The listing builds one solid part. Answer for the finished solid, in the listing's coordinates (mm). Face numbers are marked on the shaded views. A direction names the side the tool comes from. Round coordinates to 2 decimals unless told otherwise and drop trailing zeros. Write each loop counter-clockwise with the first axis right and the second up, starting at its lowest first coordinate (ties: lowest second). Pieces come first, ordered by that corner, then holes.
Item 1: Find section D-D on x = 0.2. Give the vertices of the cut face in (y, z) (3 decimals).
Item 2: Each of these flat-tipped pins is pushed along its axis until it touches: pin 1 (0.8 mm diameter, centred on y = -0.5, z = 1, fed in from -X); pin 2 (0.8 mm diameter, centred on y = -2.5, z = 1, fed in from +X); pin 3 (0.8 mm diameter, centred on x = 1.5, z = 1, fed in from -Y). Where does it stop, or does it pass through?
Item 3: Find the intervals of material crossed by probe 1 along X at (y, z) = (-4.55, 1.25); probe 2 along X at (y, z) = (-2.25, -0.05); probe 3 along Y at (x, z) = (-1.95, 1.45), in increasing order.
Item 4: Find section B-B on z = 1.6. Give the vertices of the cut face in (x, y).
Item 5: Find section C-C on y = 0.5. Give the vertices of the cut face in (x, z) (3 decimals).
Item 6: Find section A-A on z = 0. Give the vertices of the cut face in (x, y), then the cut area to 3 significant figures.
Item 7: A tool of negligible diameter and unlimited length cuts with its end or side. For the marked faces 1, 2 and 3, from which of +Z, -Z, +X, -X, +Y, -Y can it reach the whole face along a straight path? Write none if from no direction.
```python
from build123d import *

# Parameters (mm, degrees)
SKETCH1_W                  = 1.5
SKETCH1_H                  = 0.75
BOSS_EXTRUDE1_DEPTH        = 1.875
BOSS_EXTRUDE1_DEPTH_BACK   = 0.625
FILLET1_R                  = 0.5
F_0_4_0_4_DIAMETER_HOLE1_D = 0.4


with BuildPart() as part:
    # Sketch1 → Boss-Extrude1 (new body, two sides)
    with BuildSketch(Plane.XY) as boss_extrude1_sk:
        Polygon((0.285769435, 0.25), (-1.464230565, 0.25), (-1.464230565, -4), (-1.464230565, -4.75), (0.285769435, -4.75), align=None)
        Polygon((-1.464230565, 2), (-1.464230565, 0.25), (0.285769435, 0.25), (1.535769435, 0.25), (1.535769435, 2), align=None)
        with Locations((-2.214230565, -4.375)):
            Rectangle(SKETCH1_W, SKETCH1_H)
    extrude(amount=BOSS_EXTRUDE1_DEPTH)
    extrude(boss_extrude1_sk.sketch, amount=-BOSS_EXTRUDE1_DEPTH_BACK)

    # Fillet1
    fillet1_edges = [part.edges().sort_by_distance(p)[0] for p in [
        (0.285769435, 0.25, 0.625),
        (-2.964230565, -4, 0.625),
        (-1.464230565, -4, 0.625),
        (0.285769435, -4.75, 0.625),
        (-1.464230565, 2, 0.625),
    ]]
    fillet(fillet1_edges, radius=FILLET1_R)

    # Ø0.4 (0.4) Diameter Hole1 (through all)
    with Locations(Plane(origin=(0, -4, 0), x_dir=(1, 0, 0), z_dir=(0, 1, 0))):
        with Locations((-2.214230565, 0), (-2.214230565, -1.25)):
            Hole(F_0_4_0_4_DIAMETER_HOLE1_D / 2)


solid = part.part
```
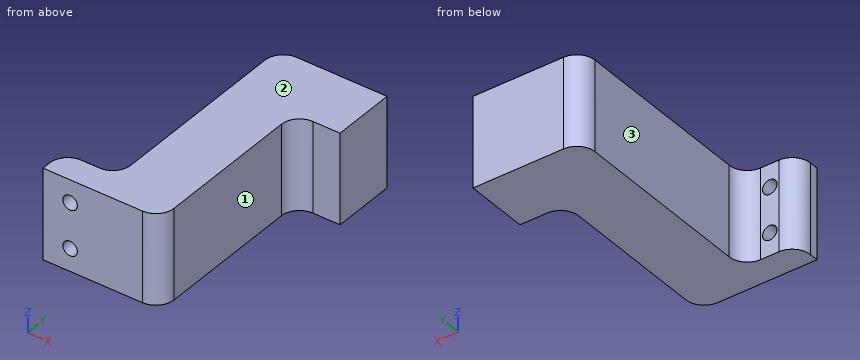
Check values:
1. outline: (-4.53, -0.625) - (2, -0.625) - (2, 1.875) - (-4.53, 1.875) - close
2. pin 1: stops at x = -1.46
2. pin 2: stops at x = 0.29
2. pin 3: stops at y = 0.25
3. probe 1: x = -2.96 to -2.41, -2.01 to 0.19
3. probe 2: x = -1.46 to 0.29
3. probe 3: y = -4.75 to -4
4. outline: (-2.96, -4.75) - (-0.21, -4.75) arc R0.5 ccw to (0.29, -4.25) - (0.29, -0.25) arc R0.5 cw to (0.79, 0.25) - (1.54, 0.25) - (1.54, 2) - (-0.96, 2) arc R0.5 ccw to (-1.46, 1.5) - (-1.46, -3.5) arc R0.5 cw to (-1.96, -4) - (-2.46, -4) arc R0.5 ccw to (-2.96, -4.5) - close
5. outline: (-1.464, -0.625) - (1.536, -0.625) - (1.536, 1.875) - (-1.464, 1.875) - close
6. outline: (-2.96, -4.75) - (-2.41, -4.75) - (-2.41, -4) - (-2.46, -4) arc R0.5 ccw to (-2.96, -4.5) - close; (-2.01, -4.75) - (-0.21, -4.75) arc R0.5 ccw to (0.29, -4.25) - (0.29, -0.25) arc R0.5 cw to (0.79, 0.25) - (1.54, 0.25) - (1.54, 2) - (-0.96, 2) arc R0.5 ccw to (-1.46, 1.5) - (-1.46, -3.5) arc R0.5 cw to (-1.96, -4) - (-2.01, -4) - close
6. area: 14.8 mm2
7. face 1: +Z, -Z, +X, -Y
7. face 2: +Z, +X, -X, +Y, -Y
7. face 3: +Z, -Z, -X, +Y
